The model under review builds one solid part; all positions refer to its coordinate system, in mm. Face numbers are marked on the shaded views. A direction names the side the tool comes from. Give positions to 0.01 mm unless a question says otherwise; leave off trailing zeros. Loops run counter-clockwise (first coordinate to the right, second up) from the corner with the lowest first, then second, coordinate; pieces in that order, holes last. Notation, with made-up numbers: M 85.25,77 L 104.25,77 A25 ccw 104.25,99 Z; hole C 39.25,44 d2. An arc over 180 degrees is marked long. Write item = value, one per line. Start each with the question number.
1. We need section C-C on y = -28. Give the boundary of the cut face in (x, z), then the cut area to 3 significant figures.
2. For the marked faces 4 and 5, list the 3-axis set-ups (+Z, -Z, +X, -X, +Y, -Y) from which the entire face can be reached by the end or side of a thin tool; tool diameter is ignored.
3. We need section A-A on x = -10. Give the boundary of the cut face in (y, z), then the cut area to 4 significant figures.
4. Draft analysis for pull direction Y (two halves, no side actions). For the marked faces 1, 2 and 3, state which applies: pulls with the +Y half, pulls with the -Y half, needs draft (parallel to the pull), parting line crosses it, or undercut.
5. We need section D-D on z = 59.8. Count the separate pieces of the cut face and the enclosed holes in it, then the cut area to 3 significant figures.
6. For pin 1 (5 mm diameter, centred on x = -57, y = -33, fed in from +Z); pin 2 (4.5 mm diameter, centred on x = -2.5, y = -21.5, fed in from +Z); pin 3 (1.8 mm diameter, centred on x = -19.49, z = 47.99, fed in from +Y), all flat-tipped, find the tip position at first contact; note any pin that passes through.
7. Wall thickness on line 1 along Y through (x, z) = (-103, 101); line 2 along X through (y, z) = (-33, 43.5); line 3 along Z through (x, y) = (-102, -56): over which ranges is each line inside the solid? List them lowest first. Write a range as from..to.
8. We need section B-B on z = 91. Give the boundary of the cut face in (x, y), then the cut area to 3 significant figures.
from build123d import *

# Parameters (mm, degrees)
F7_W      = 57
F7_H      = 65
F8_DEPTH  = 3
F6_W      = 114
F6_H      = 57
F6_W_2    = 30
F6_H_2    = 10
F9_DEPTH  = 2
F10_R     = 4.99999
F5_W      = 57
F5_H      = 53.4
F5_R      = 1.8
F11_DEPTH = 4
F12_W     = 51
F12_H     = 25.25
F13_DEPTH = 1.1
F14_DEPTH = 4
F15_W     = 5
F15_H     = 25.25
F16_DEPTH = 4.1
F1_W      = 111
F1_H      = 65
F1_R      = 1.5
F1_W_2    = 8
F1_H_2    = 8
F1_R_2    = 1.6
F1_R_3    = 2.1
F17_DEPTH = 2
F19_SIZE  = 2
F20_SIZE  = 2
F18_W     = 111
F18_H     = 65
F18_R     = 1.8
F18_W_2   = 28.2
F18_H_2   = 22
F21_DEPTH = 4
F22_SIZE  = 2
F23_SIZE  = 2
F24_SIZE  = 0.99999
F25_SIZE  = 0.99999
F26_R     = 0.5
F27_W     = 1.2
F27_H     = 4
F28_DEPTH = 22
F29_SIZE  = 0.6
F31_DEPTH = 1.3
F33_DEPTH = 2.38
F35_DEPTH = 1.2
F36_W     = 8
F36_H     = 8
F37_DEPTH = 2.6


# Not quite as in the source:
# - a fillet or chamfer is up to 0.001 mm smaller than in the source, because OpenCascade refuses the exact size


with BuildPart() as f8:
    # F7 (on offset) → F8 (new body)
    with BuildSketch(Plane.YZ.offset(-111)):
        with Locations((-28.5, 72.5)):
            Rectangle(F7_W, F7_H)
    extrude(amount=-F8_DEPTH)

    # F6 (on offset) → F9 (join)
    with BuildSketch(Plane.XY.offset(40)):
        with Locations((-57, -28.5)):
            Rectangle(F6_W, F6_H)
        with Locations((-40, -20)):
            Rectangle(F6_W_2, F6_H_2, mode=Mode.SUBTRACT)
    extrude(amount=-F9_DEPTH)

    # F10 (radius 5 in the source; OpenCascade refuses exactly that, so slightly less here)
    f10_edges = [f8.edges().sort_by_distance(p)[0] for p in [
        (-25, -25, 39),
        (-55, -25, 39),
        (-55, -15, 39),
        (-25, -15, 39),
    ]]
    fillet(f10_edges, radius=F10_R)

    # F5 (on Right) → F11 (join)
    with BuildSketch(Plane.YZ):
        with Locations((-28.5, 66.7)):
            Rectangle(F5_W, F5_H)
        with Locations((-46.4825592935, 85.7889130712)):
            Circle(F5_R, mode=Mode.SUBTRACT)
        with Locations((-36.4768356085, 85.8261138201)):
            Circle(F5_R, mode=Mode.SUBTRACT)
    extrude(amount=-F11_DEPTH)

    # F12 (on face) → F13 (cut)
    with BuildSketch(Plane.YZ):
        with Locations((-27.5, 92.375)):
            Rectangle(F12_W, F12_H)
    extrude(amount=-F13_DEPTH, mode=Mode.SUBTRACT)

    # F14 (add): a face of the model
    f14_faces = [f8.faces().sort_by_distance(p)[0] for p in [
        (0, -28.7827981232, 59.796589178),
    ]]
    extrude(f14_faces, amount=-F14_DEPTH)

    # F15 (on face) → F16 (cut)
    with BuildSketch(Plane.YZ):
        with Locations((-4.5, 92.375)):
            Rectangle(F15_W, F15_H)
    extrude(amount=-F16_DEPTH, mode=Mode.SUBTRACT)

    # F1 (on offset) → F17 (join)
    with BuildSketch(Plane.XZ.offset(2)):
        with Locations((-55.5, 72.5)):
            Rectangle(F1_W, F1_H)
        with Locations((-93.9863845706, 48.0133742094)):
            Circle(F1_R, mode=Mode.SUBTRACT)
        with Locations((-19.4850880653, 47.9871667922)):
            Circle(F1_R, mode=Mode.SUBTRACT)
        with Locations((-7.9999973103, 68.4999966025)):
            Rectangle(F1_W_2, F1_H_2, mode=Mode.SUBTRACT)
        with Locations((-103.55, 84.9350020289)):
            Circle(F1_R_2, mode=Mode.SUBTRACT)
        with Locations((-6.4611095004, 84.4112932682)):
            Circle(F1_R_3, mode=Mode.SUBTRACT)
    extrude(amount=-F17_DEPTH)

    # F19
    f19_edges = [f8.edges().sort_by_distance(p)[0] for p in [
        (0, 0, 71.5),
    ]]
    chamfer(f19_edges, length=F19_SIZE)

    # F20
    f20_edges = [f8.edges().sort_by_distance(p)[0] for p in [
        (-114, 0, 71.5),
    ]]
    chamfer(f20_edges, length=F20_SIZE)

    # F18 (on offset) → F21 (join)
    with BuildSketch(Plane.XZ.offset(53)):
        with Locations((-55.5, 72.5)):
            Rectangle(F18_W, F18_H)
        with Locations((-102, 59.8)):
            Circle(F18_R, mode=Mode.SUBTRACT)
        Polygon((-96, 64.2), (-90.6, 69.6), (-73.4, 69.6), (-68, 64.2), (-68, 50), (-96, 50), align=None, mode=Mode.SUBTRACT)
        with Locations((-62, 59.8)):
            Circle(F18_R, mode=Mode.SUBTRACT)
        with Locations((-33.1, 59.8)):
            Rectangle(F18_W_2, F18_H_2, mode=Mode.SUBTRACT)
    extrude(amount=F21_DEPTH)

    # F22
    f22_edges = [f8.edges().sort_by_distance(p)[0] for p in [
        (0, -57, 71.5),
    ]]
    chamfer(f22_edges, length=F22_SIZE)

    # F23
    f23_edges = [f8.edges().sort_by_distance(p)[0] for p in [
        (-114, -57, 71.5),
    ]]
    chamfer(f23_edges, length=F23_SIZE)

    # F24 (size 1 in the source; OpenCascade refuses exactly that, so slightly less here)
    f24_edges = [f8.edges().sort_by_distance(p)[0] for p in [
        (-57, -57, 105),
        (-57, 0, 105),
        (-114, -28.5, 105),
    ]]
    chamfer(f24_edges, length=F24_SIZE)

    # F25 (size 1 in the source; OpenCascade refuses exactly that, so slightly less here)
    f25_edges = [f8.edges().sort_by_distance(p)[0] for p in [
        (-57, -57, 38),
        (-114, -28.5, 38),
    ]]
    chamfer(f25_edges, length=F25_SIZE)

    # F26
    f26_edges = [f8.edges().sort_by_distance(p)[0] for p in [
        (-40, -25, 38),
        (-53.535537, -23.535537, 38),
        (-40, -15, 38),
        (-26.464463, -16.464463, 38),
        (-26.464463, -16.464463, 40),
        (-53.535537, -23.535537, 40),
    ]]
    fillet(f26_edges, radius=F26_R)

    # F27 (on face) → F28 (join, through all)
    with BuildSketch(Plane.XY.offset(48.8)):
        with Locations((-33.1, -55)):
            Rectangle(F27_W, F27_H)
        with Locations((-40.6, -55)):
            Rectangle(F27_W, F27_H)
        with Locations((-25.6, -55)):
            Rectangle(F27_W, F27_H)
    extrude(amount=F28_DEPTH)

    # F29
    f29_edges = [f8.edges().sort_by_distance(p)[0] for p in [
        (-82, -57, 50),
        (-68, -57, 57.1),
        (-70.7, -57, 66.9),
        (-82, -57, 69.6),
        (-93.3, -57, 66.9),
        (-96, -57, 57.1),
    ]]
    chamfer(f29_edges, length=F29_SIZE)

    # F30 (on face) → F31 (cut)
    with BuildSketch(Plane(origin=(-4, 0, 0), x_dir=(0, -1, 0), z_dir=(-1, 0, 0))):
        Polygon((39.1768356085, 84.2672680933), (39.1768356085, 87.3849595469), (36.4768356085, 88.9438052737), (33.7768356085, 87.3849595469), (33.7768356085, 84.2672680933), (36.4768356085, 82.7084223665), align=None)
        Polygon((49.1825592935, 84.2300673443), (49.1825592935, 87.347758798), (46.4825592935, 88.9066045248), (43.7825592935, 87.347758798), (43.7825592935, 84.2300673443), (46.4825592935, 82.6712216175), align=None)
    extrude(amount=-F31_DEPTH, mode=Mode.SUBTRACT)

    # F32 (on face) → F33 (cut)
    with BuildSketch(Plane.XZ.offset(53)):
        Polygon((-64.7, 61.3588457268), (-64.7, 58.2411542732), (-62, 56.6823085464), (-59.3, 58.2411542732), (-59.3, 61.3588457268), (-62, 62.9176914536), align=None)
        Polygon((-104.7, 61.3588457268), (-104.7, 58.2411542732), (-102, 56.6823085464), (-99.3, 58.2411542732), (-99.3, 61.3588457268), (-102, 62.9176914536), align=None)
    extrude(amount=F33_DEPTH, mode=Mode.SUBTRACT)

    # F34 (on face) → F35 (cut)
    with BuildSketch(Plane.XZ.offset(2)):
        Polygon((-91.2863845706, 46.4545284826), (-91.2863845706, 49.5722199362), (-93.9863845706, 51.131065663), (-96.6863845706, 49.5722199362), (-96.6863845706, 46.4545284826), (-93.9863845706, 44.8956827558), align=None)
        Polygon((-16.7850880653, 46.4283210653), (-16.7850880653, 49.546012519), (-19.4850880653, 51.1048582458), (-22.1850880653, 49.546012519), (-22.1850880653, 46.4283210653), (-19.4850880653, 44.8694753385), align=None)
    extrude(amount=-F35_DEPTH, mode=Mode.SUBTRACT)

    # F36 (on face) → F37 (cut)
    with BuildSketch(Plane.YZ):
        with Locations((-40, 50.8261138201)):
            Rectangle(F36_W, F36_H)
    extrude(amount=-F37_DEPTH, mode=Mode.SUBTRACT)


solid = f8.part
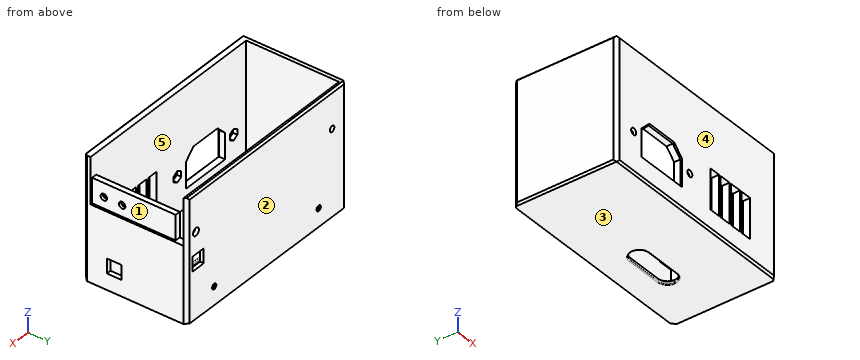
Final values:
q1.outline = M -114,39 L -113,38 L 0,38 L 0,79.75 L -1.1,79.75 L -1.1,93.4 L -4,93.4 L -4,40 L -111,40 L -111,105 L -113,105 L -114,104 Z
q1.area = 621 mm²
q2.face_4 = +Z, -Z, +X, -X, -Y
q2.face_5 = +Z
q3.outline = M -57,39 L -56,38 L 0,38 L 0,64.5 L -2,64.5 L -2,40 L -53,40 L -53,105 L -56,105 L -57,104 Z; M -2,72.5 L 0,72.5 L 0,104 L -1,105 L -2,105 Z
q3.area = 486.5 mm²
q4.face_1 = undercut
q4.face_2 = pulls with the +Y half
q4.face_3 = needs draft
q5.separate_pieces = 7
q5.enclosed_holes = 0
q5.area = 785 mm²
q6.pin_1 = 40
q6.pin_2 = 93.4
q6.pin_3 = -53
q7.line_1 = -57..-53, -2..0
q7.line_2 = -114..-111, -4..0
q7.line_3 = 38..58, 61.6..105
q8.outline = M -114,-55 L -112,-57 L -2,-57 L 0,-55 L 0,-53 L -1.1,-53 L -1.1,-7 L -4,-7 L -4,-53 L -111,-53 L -111,-2 L 0,-2 L -2,0 L -112,0 L -114,-2 Z
q8.area = 962 mm²
